from build123d import *

# Parameters (mm, degrees)
SKETCH3_W           = 690
SKETCH3_H           = 1970
BOSS_EXTRUDE2_DEPTH = 20
SKETCH4_W           = 440
SKETCH4_H           = 1970
CUT_EXTRUDE1_DEPTH  = 5
SKETCH5_W           = 440
SKETCH5_H           = 5
CUT_EXTRUDE2_DEPTH  = 16
SKETCH6_W           = 440
SKETCH6_H           = 320
CUT_EXTRUDE8_DEPTH  = 10
SKETCH7_W           = 5
SKETCH7_H           = 320
CUT_EXTRUDE9_DEPTH  = 5
SKETCH8_W           = 30
SKETCH8_H           = 240
CUT_EXTRUDE10_DEPTH = 5
CUT_EXTRUDE11_DEPTH = 3


with BuildPart() as part:
    # Sketch3 → Boss-Extrude2 (new body)
    with BuildSketch(Plane.XY):
        with Locations((345, -985)):
            Rectangle(SKETCH3_W, SKETCH3_H)
    boss_extrude2 = extrude(amount=-BOSS_EXTRUDE2_DEPTH)

    # Sketch4 → Cut-Extrude1 (cut)
    with BuildSketch(Plane.XY):
        with Locations((345, -985)):
            Rectangle(SKETCH4_W, SKETCH4_H)
    cut_extrude1 = extrude(amount=-CUT_EXTRUDE1_DEPTH, mode=Mode.SUBTRACT)

    # Sketch5 → Cut-Extrude2 (cut, through all)
    with BuildSketch(Plane.XY.offset(-5)):
        with Locations((345, -2.5)):
            Rectangle(SKETCH5_W, SKETCH5_H)
        with Locations((345, -1967.5)):
            Rectangle(SKETCH5_W, SKETCH5_H)
    cut_extrude2 = extrude(amount=-CUT_EXTRUDE2_DEPTH, mode=Mode.SUBTRACT)

    # Sketch6 → Cut-Extrude8 (cut)
    with BuildSketch(Plane.XY):
        with Locations((345, -485)):
            Rectangle(SKETCH6_W, SKETCH6_H)
        with Locations((345, -985)):
            Rectangle(SKETCH6_W, SKETCH6_H)
        with Locations((345, -1485)):
            Rectangle(SKETCH6_W, SKETCH6_H)
    cut_extrude8 = extrude(amount=-CUT_EXTRUDE8_DEPTH, mode=Mode.SUBTRACT)

    # Sketch7 → Cut-Extrude9 (cut)
    with BuildSketch(Plane.XY.offset(-10)):
        with Locations((427.5, -485)):
            Rectangle(SKETCH7_W, SKETCH7_H)
        with Locations((262.5, -985)):
            Rectangle(SKETCH7_W, SKETCH7_H)
        with Locations((427.5, -1485)):
            Rectangle(SKETCH7_W, SKETCH7_H)
    cut_extrude9 = extrude(amount=-CUT_EXTRUDE9_DEPTH, mode=Mode.SUBTRACT)

    # Mirror1: Boss-Extrude2, Cut-Extrude1, Cut-Extrude2, Cut-Extrude8, Cut-Extrude9 across plane
    add(boss_extrude2.mirror(Plane.XY.offset(-20)))
    add(cut_extrude1.mirror(Plane.XY.offset(-20)), mode=Mode.SUBTRACT)
    add(cut_extrude2.mirror(Plane.XY.offset(-20)), mode=Mode.SUBTRACT)
    add(cut_extrude8.mirror(Plane.XY.offset(-20)), mode=Mode.SUBTRACT)
    add(cut_extrude9.mirror(Plane.XY.offset(-20)), mode=Mode.SUBTRACT)

    # Sketch8 → Cut-Extrude10 (cut)
    with BuildSketch(Plane(origin=(690, 0, 0), x_dir=(0, 0, -1), z_dir=(1, 0, 0))):
        with Locations((20, -1025)):
            Rectangle(SKETCH8_W, SKETCH8_H)
    extrude(amount=-CUT_EXTRUDE10_DEPTH, mode=Mode.SUBTRACT)

    # Sketch9 → Cut-Extrude11 (cut)
    with BuildSketch(Plane.ZY):
        with BuildLine():
            Line((-35, -400), (-35, -490))
            ThreePointArc((-35, -490), (-20, -500), (-5, -490))
            Line((-5, -490), (-5, -450))
            Line((-5, -450), (0, -450))
            Line((0, -450), (0, -400))
            Line((0, -400), (-35, -400))
        make_face()
        with BuildLine():
            Line((-35, -1790), (-35, -1880))
            ThreePointArc((-35, -1880), (-20, -1890), (-5, -1880))
            Line((-5, -1880), (-5, -1840))
            Line((-5, -1840), (0, -1840))
            Line((0, -1840), (0, -1790))
            Line((0, -1790), (-35, -1790))
        make_face()
    extrude(amount=-CUT_EXTRUDE11_DEPTH, mode=Mode.SUBTRACT)


solid = part.part
Check sheet for the modelled part. Datum: model origin and axes. Units: mm. A direction names the side the tool comes from. Round coordinates to 2 decimals unless told otherwise and drop trailing zeros. Order: outer loops, then holes, each group sorted by start corner. A loop starts at its lowest first (then second) coordinate and runs counter-clockwise, first axis right, second up.
Q1. Cross-section at A-A, the plane y = -170. Enter the section's corners in (x, z), plus the area to 3 significant figures.
Filled sheet:
outline: (0, -40) - (125, -40) - (125, -35) - (565, -35) - (565, -40) - (690, -40) - (690, 0) - (565, 0) - (565, -5) - (125, -5) - (125, 0) - (0, 0) - close
area: 23,200 mm2
Q2. Scan lines: L1, parallel to Y at x = 250.5, z = -9; L2, parallel to X at y = -342, z = -7; L3, parallel to Y at x = 413, z = -15. Record each from-to range of solid material in increasing order.
Filled sheet:
L1: y = -1965 to -1645, -1325 to -1145, -825 to -645, -325 to -5
L2: x = 0 to 125, 565 to 690
L3: y = -1965 to -5
Q3. Draft check along Y on faces 1 (the face through (62, -1970, -20)), 2 (the face through (565, -990, -8)), 3 (the face through (342, -1234, -35)), 4 (the face through (413, -983, -30)). Enter one of: pulls with the +Y half, pulls with the -Y half, needs draft (parallel to the pull), parting line crosses it, or undercut.
Filled sheet:
face 1: pulls with the -Y half
face 2: undercut
face 3: needs draft
face 4: undercut
Q4. Set-up check for faces 5 (the face through (342, -163, -5)), 6 (the face through (497, -1483, -10)), 7 (the face through (125, -990, -8)), 8 (the face through (497, -1483, -30)): record each of +Z, -Z, +X, -X, +Y, -Y from which the full face is reachable in a straight line by a thin tool's end or side.
Filled sheet:
face 5: +Z, +Y, -Y
face 6: +Z
face 7: none
face 8: -Z
Q5. Cross-section at B-B, the plane x = 307.5. Enter the section's corners in (y, z).
Filled sheet:
outline: (-1965, -35) - (-1645, -35) - (-1645, -30) - (-1325, -30) - (-1325, -35) - (-1145, -35) - (-1145, -30) - (-825, -30) - (-825, -35) - (-645, -35) - (-645, -30) - (-325, -30) - (-325, -35) - (-5, -35) - (-5, -5) - (-325, -5) - (-325, -10) - (-645, -10) - (-645, -5) - (-825, -5) - (-825, -10) - (-1145, -10) - (-1145, -5) - (-1325, -5) - (-1325, -10) - (-1645, -10) - (-1645, -5) - (-1965, -5) - close
Q6. Cross-section at D-D, the plane y = -1413. Enter the section's corners in (x, z), plus the area to 4 significant figures.
Filled sheet:
outline: (0, -40) - (125, -40) - (125, -30) - (425, -30) - (425, -25) - (430, -25) - (430, -30) - (565, -30) - (565, -40) - (690, -40) - (690, 0) - (565, 0) - (565, -10) - (430, -10) - (430, -15) - (425, -15) - (425, -10) - (125, -10) - (125, 0) - (0, 0) - close
area: 18,750 mm2
Q7. Cross-section at C-C, the plane y = -1041. Enter the section's corners in (x, z).
Filled sheet:
outline: (0, -40) - (125, -40) - (125, -30) - (260, -30) - (260, -25) - (265, -25) - (265, -30) - (565, -30) - (565, -40) - (690, -40) - (690, -35) - (685, -35) - (685, -5) - (690, -5) - (690, 0) - (565, 0) - (565, -10) - (265, -10) - (265, -15) - (260, -15) - (260, -10) - (125, -10) - (125, 0) - (0, 0) - close
Q8. Depth check by flat-ended pin: P1, Ø3, axis at x = 383, z = -9, coming from the +Y side; P2, Ø5.5, axis at x = 427, y = -1493, coming from the +Z side; P3, Ø10, axis at x = 304, z = -11, coming from the -Y side. Enter the tip coordinate at first touch or a pass-through.
Filled sheet:
P1: stops at y = -5
P2: stops at z = -10
P3: stops at y = -1965
